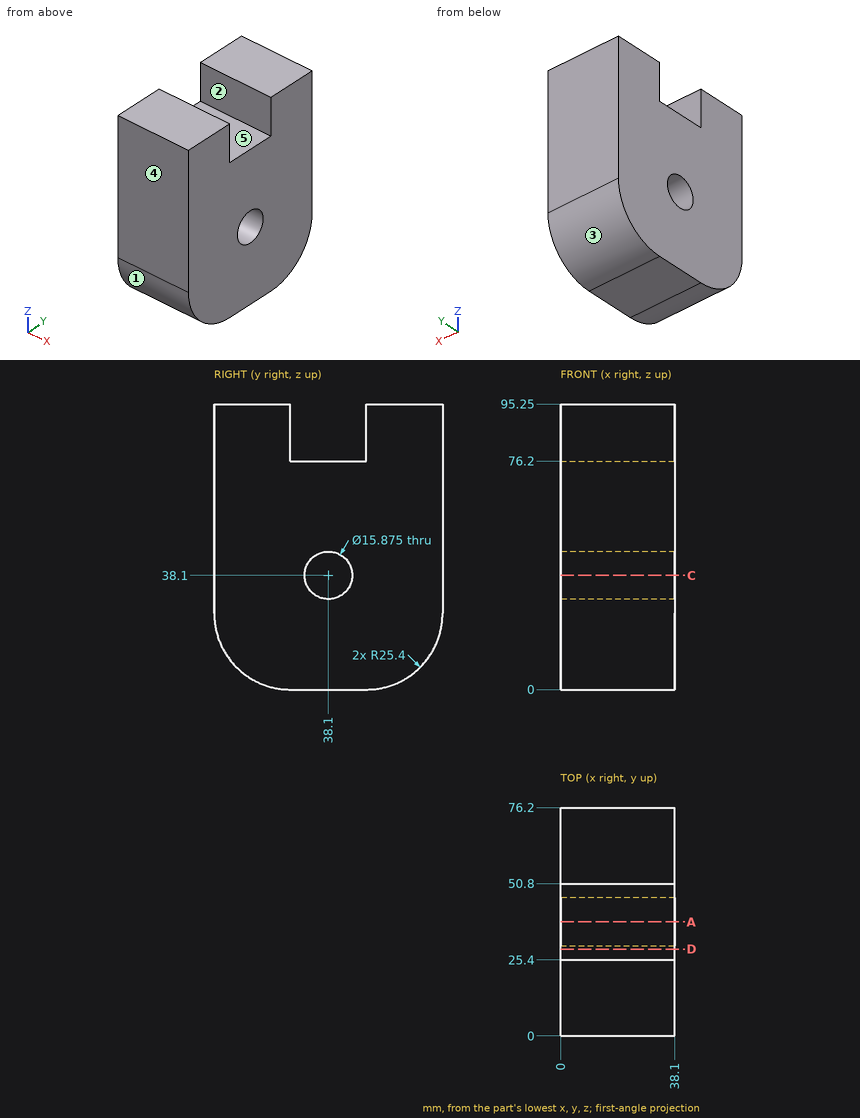
Check sheet for the drawn part. Datum: minimum x, y, z corner. Units: mm. A direction names the side the tool comes from. Round coordinates to 2 decimals unless told otherwise and drop trailing zeros. Loops run counter-clockwise (first coordinate to the right, second up) from the corner with the lowest first, then second, coordinate; pieces in that order, holes last. Notation, with made-up numbers: (-36.75, 66.5) -> (-12.75, 66.5) arc R25 cw to (-12.75, 101.5) -> close; hole circle Ø10 at (54.5, -8.5). An arc over 180 degrees is marked (long way). Put each result on its own line as item: value. Start each with the question number.
1. Section check D-D (y = 29). Enter the section's corners in (x, z), plus the area to 3 significant figures.
2. Section check A-A (y = 38.1). Enter the section's corners in (x, z), plus the area to 3 significant figures.
3. Draft check along Y on the marked faces 1, 2 and 3. Enter one of: +Y half, -Y half, draft (parallel to the pull), parting line (faces both ways), or undercut.
4. Gauge pin test, flat ends, axial feed: pin 1 (4 mm diameter, centred on x = 26, y = 10, fed in from -Z); pin 2 (7.5 mm diameter, centred on x = 13.5, y = 35, fed in from +Z). Record the tip position at first contact, or that the pin passes through.
5. Access from +Z, -Z, +X, -X, +Y, -Y to the whole of each face (thin tool, end or side, straight path). Record for the marked faces 4 and 5.
6. Scan lines: probe 1 along Z at (x, y) = (27.5, 38.1); probe 2 along Z at (x, y) = (9, 50). Record each from-to range of solid material in increasing order.
Findings:
1. outline: (0, 0) -> (38.1, 0) -> (38.1, 76.2) -> (0, 76.2) -> close
1. area: 2,900 mm^2
2. outline: (0, 0) -> (38.1, 0) -> (38.1, 30.16) -> (0, 30.16) -> close; (0, 46.04) -> (38.1, 46.04) -> (38.1, 76.2) -> (0, 76.2) -> close
2. area: 2,300 mm^2
3. face 1: -Y half
3. face 2: undercut
3. face 3: +Y half
4. pin 1: stops at z = 3.82
4. pin 2: stops at z = 76.2
5. face 4: +Z, -Z, +X, -X, -Y
5. face 5: +Z, +X, -X
6. probe 1: z = 0 to 30.16, 46.04 to 76.2
6. probe 2: z = 0 to 76.2
